Input: part model. Units: mm. Frame: model coordinates. Face numbers are marked on the shaded views. A direction names the side the tool comes from. Coordinates: 2 decimals unless noted, no trailing zeros. Order: outer loops, then holes, each group sorted by start corner. A loop starts at its lowest first (then second) coordinate and runs counter-clockwise, first axis right, second up. Notation, with made-up numbers: (85, 17.5) -> (99, 17.5) arc R9 ccw to (99, 25.5) -> close; hole circle Ø9 at (24, -23). An arc over 180 degrees is marked (long way). Use CSV: the item, a comma, the result in double quotes. Start each with the question number.
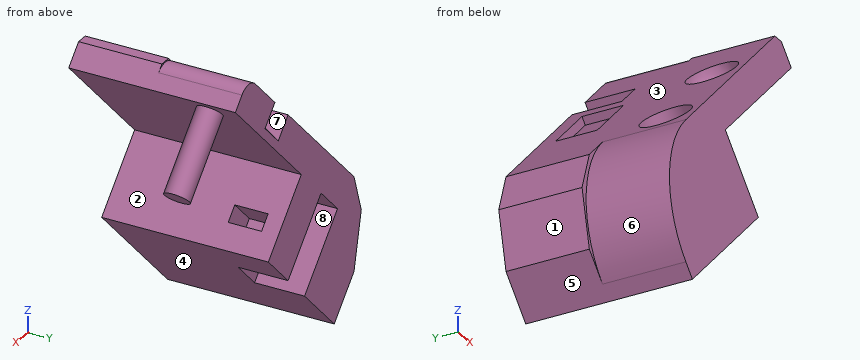
```python
from build123d import *

# Parameters (mm, degrees)
SKICA1_W                 = 200
SKICA1_H                 = 100
P_IDAT_VYSUNUT_M1_DEPTH  = 20
P_IDAT_VYSUNUT_M2_DEPTH  = 50
SKICA7_R                 = 7.5
P_IDAT_VYSUNUT_M3_DEPTH  = 50
ODEBRAT_VYSUNUT_M3_DEPTH = 10
ZAOBLIT1_START           = 50
ZAOBLIT1_DEPTH           = 51
SKICA9_W                 = 40
SKICA9_H                 = 25
ODEBRAT_VYSUNUT_M4_DEPTH = 5
CHAMFER2_SIZE            = 5
FILLET2_DEPTH            = 50
CHAMFER3_SIZE            = 40
CHAMFER3_SIZE2           = 20
CHAMFER4_SIZE            = 20
SKETCH3_R                = 15
CUT_EXTRUDE2_DEPTH       = 60
SKETCH4_W                = 10
SKETCH4_H                = 20
CUT_EXTRUDE3_DEPTH       = 22


with BuildPart() as part:
    # Skica1 → Přidat vysunutím1 (new body)
    with BuildSketch(Plane(origin=(0, 0, 0), x_dir=(-0.7071067811865476, 0, -0.7071067811865476), z_dir=(0.7071067811865476, 0, -0.7071067811865476))):
        with Locations((100, 50)):
            Rectangle(SKICA1_W, SKICA1_H)
    extrude(amount=P_IDAT_VYSUNUT_M1_DEPTH)

    # Skica2 → Přidat vysunutím2 (add)
    with BuildSketch(Plane(origin=(14.142135624, 0, -14.142135624), x_dir=(-0.7071067811865478, 0, -0.7071067811865472), z_dir=(0.7071067811865472, 0, -0.7071067811865478))):
        Polygon((100, 0), (200, 0), (200, 100), (155, 100), (155, 70), (130, 70), (130, 100), (100, 100), align=None)
    extrude(amount=P_IDAT_VYSUNUT_M2_DEPTH)

    # Skica7 → Přidat vysunutím3 (add)
    with BuildSketch(Plane(origin=(14.142135624, 0, -14.142135624), x_dir=(-0.7071067811865478, 0, -0.7071067811865472), z_dir=(0.7071067811865472, 0, -0.7071067811865478))):
        with Locations(Location((12, 80, 0), (0, 0, 180))):
            Circle(SKICA7_R)
    extrude(amount=P_IDAT_VYSUNUT_M3_DEPTH)

    # Skica8 → Odebrat vysunutím3 (cut, symmetric)
    with BuildSketch(Plane(origin=(-35.355339059, 0, -35.355339059), x_dir=(0.7071067811865476, 0, -0.7071067811865475), z_dir=(0.7071067811865475, 0, 0.7071067811865476))):
        Polygon((0, 100), (0, 70), (15, 100), align=None)
    extrude(amount=ODEBRAT_VYSUNUT_M3_DEPTH, both=True, mode=Mode.SUBTRACT)

    # Zaoblit1: read off the stored shape, not the designer's step
    # Zaoblit1 outline → Zaoblit1 (cut)
    with BuildSketch(Plane(origin=(0, 0, 0), x_dir=(1, 0, 0), z_dir=(0, 1, 0)).offset(ZAOBLIT1_START)):
        with BuildLine():
            ThreePointArc((7.071067812, 7.071067812), (0, 4.142135624), (-7.071067812, 7.071067812))
            Line((-7.071067812, 7.071067812), (0, 0))
            Line((0, 0), (7.071067812, 7.071067812))
        make_face()
    extrude(amount=ZAOBLIT1_DEPTH, mode=Mode.SUBTRACT)

    # Skica9 → Odebrat vysunutím4 (cut)
    with BuildSketch(Plane(origin=(0, 0, 0), x_dir=(0.7071067811865478, 0, 0.7071067811865472), z_dir=(-0.7071067811865472, 0, 0.7071067811865478))):
        with Locations((-90, 77.5)):
            Rectangle(SKICA9_W, SKICA9_H)
    extrude(amount=-ODEBRAT_VYSUNUT_M4_DEPTH, mode=Mode.SUBTRACT)

    # Chamfer2
    chamfer2_edges = [part.edges().sort_by_distance(p)[0] for p in [
        (0, 25, 0),
    ]]
    chamfer(chamfer2_edges, length=CHAMFER2_SIZE)

    # Fillet2: read off the stored shape, not the designer's step
    # Fillet2 outline → Fillet2 (cut)
    with BuildSketch(Plane(origin=(0, 0, 0), x_dir=(1, 0, 0), z_dir=(0, 1, 0))):
        with BuildLine():
            Line((-141.421356237, 141.421356237), (-98.994949366, 98.994949366))
            ThreePointArc((-98.994949366, 98.994949366), (-116.568542495, 141.421356238), (-98.994949366, 183.847763109))
            Line((-98.994949366, 183.847763109), (-141.421356237, 141.421356237))
        make_face()
    extrude(amount=FILLET2_DEPTH, mode=Mode.SUBTRACT)

    # Chamfer3
    chamfer3_edges = [part.edges().sort_by_distance(p)[0] for p in [
        (-141.421356237, 75, -141.421356237),
    ]]
    chamfer3_side = [part.faces().sort_by_distance(p)[0] for p in [
        (-65.974510685, 51.38225256, -65.974510685),
    ]]
    chamfer(chamfer3_edges, length=CHAMFER3_SIZE, length2=CHAMFER3_SIZE2, reference=chamfer3_side[0])

    # Chamfer4
    chamfer4_edges = [part.edges().sort_by_distance(p)[0] for p in [
        (-127.279220614, 75, -155.563491861),
    ]]
    chamfer(chamfer4_edges, length=CHAMFER4_SIZE)

    # Sketch2 → Cut-Revolve4 (revolve, cut)
    with BuildSketch(Plane(origin=(0, 0, 0), x_dir=(0.7071067811865478, 0, 0.7071067811865472), z_dir=(-0.7071067811865472, 0, 0.7071067811865478))):
        with BuildLine():
            Line((-50, 35), (-50, 5))
            ThreePointArc((-50, 5), (-35, 20), (-50, 35))
        make_face()
    revolve(axis=Axis((-35.355339059, 35, -35.355339059), (0, -1, 0)), mode=Mode.SUBTRACT)

    # Sketch3 → Cut-Extrude2 (cut)
    with BuildSketch(Plane(origin=(0, 0, 0), x_dir=(0.7071067811865478, 0, 0.7071067811865472), z_dir=(-0.7071067811865472, 0, 0.7071067811865478))):
        with Locations((-120, 20)):
            Circle(SKETCH3_R)
    extrude(amount=-CUT_EXTRUDE2_DEPTH, mode=Mode.SUBTRACT)

    # Sketch4 → Cut-Extrude3 (cut)
    with BuildSketch(Plane(origin=(-70.710678119, 0, -70.710678119), x_dir=(0.7071067811865472, 0, -0.7071067811865478), z_dir=(0.7071067811865478, 0, 0.7071067811865472))):
        with Locations((50, 80)):
            Rectangle(SKETCH4_W, SKETCH4_H)
    extrude(amount=-CUT_EXTRUDE3_DEPTH, mode=Mode.SUBTRACT)


solid = part.part
```
1. Section A-A on y = 39.5. Return loops of the section in (x, z), then the cut area to 3 significant figures.
2. Section D-D on y = 62. Return loops of the section in (x, z).
3. Material intervals for line 1 along Z through (x, y) = (-55.5, 23.5); line 2 along X through (y, z) = (83.5, -134.5); line 3 along Z through (x, y) = (-93, 85), sorted ascending.
4. Contact query for flat-ended pins moving along their axis: P1, Ø10, axis at x = 19, y = 19, coming from the -Z side; P2, Ø1.5, axis at x = 6, y = 32, coming from the +Z side; P3, Ø2, axis at x = -83.5, y = 35.5, coming from the +Z side. Output: stop coordinate, or through.
5. Section B-B on z = -152. Return loops of the section in (x, y), then the cut area to 3 significant figures.
6. Access query for the marked faces 4, 5, 6, 7 and 8. Directions: +Z, -Z, +X, -X, +Y, -Y. A direction counts if a zero-diameter tool reaches every point of the face in a straight line with its end or side. Return the directions, or none.
7. Section C-C on y = 12. Return loops of the section in (x, z) (3 decimals).
8. Pull-direction query (Z, two-part tool) for the marked faces 1, 2 and 3; classes: released by +Z, released by -Z, zero draft, split by the parting line, or undercut.
Values follow:
1,outline,"(-98.99, -183.85) -> (-91.92, -190.92) -> (-21.21, -120.21) -> (-56.57, -84.85) -> (14.14, -14.14) -> (3.54, -3.54) -> (-3.54, -3.54) -> (-98.99, -98.99) arc R60 ccw to start"
1,area,"8,210 mm2"
2,outline,"(-120.95, -136.59) -> (-113.14, -169.71) -> (-91.92, -190.92) -> (-21.21, -120.21) -> (-56.57, -84.85) -> (14.14, -14.14) -> (7.07, -7.07) arc R10 ccw to (-7.07, -7.07) -> (-113.14, -113.14) -> close"
3,line 1,"z = -154.49 to -134.83, -93.58 to -85.92, -83.78 to -55.5"
3,line 2,"x = -120.26 to -84.7, -49.35 to -35.51"
3,line 3,"z = -189.84 to -126.2, -121.28 to -93"
4,P1,"stops at z = -14.28"
4,P2,"stops at z = -5.25"
4,P3,"stops at z = -82.5"
5,outline,"(-117.32, 50) -> (-115.63, 50) -> (-115.63, 0) -> (-53.01, 0) -> (-53.01, 70) -> (-67.2, 70) -> (-67.2, 100) -> (-117.32, 100) -> close"
5,area,"5,920 mm2"
6,face 4,"-Z, +X, +Y, -Y"
6,face 5,"-Z, -X, +Y, -Y"
6,face 6,"-X, -Y"
6,face 7,"+Z, +Y"
6,face 8,"+Y"
7,outline,"(-98.995, -183.848) -> (-91.924, -190.919) -> (-21.213, -120.208) -> (-56.569, -84.853) -> (14.142, -14.142) -> (3.536, -3.536) -> (-3.536, -3.536) -> (-26.383, -26.383) arc R12.689 cw to (-44.328, -44.328) -> (-75.881, -75.881) -> (-33.454, -118.307) -> (-51.399, -136.251) -> (-93.825, -93.825) -> (-98.995, -98.995) arc R60 ccw to start"
8,face 1,"released by -Z"
8,face 2,"undercut"
8,face 3,"released by +Z"
